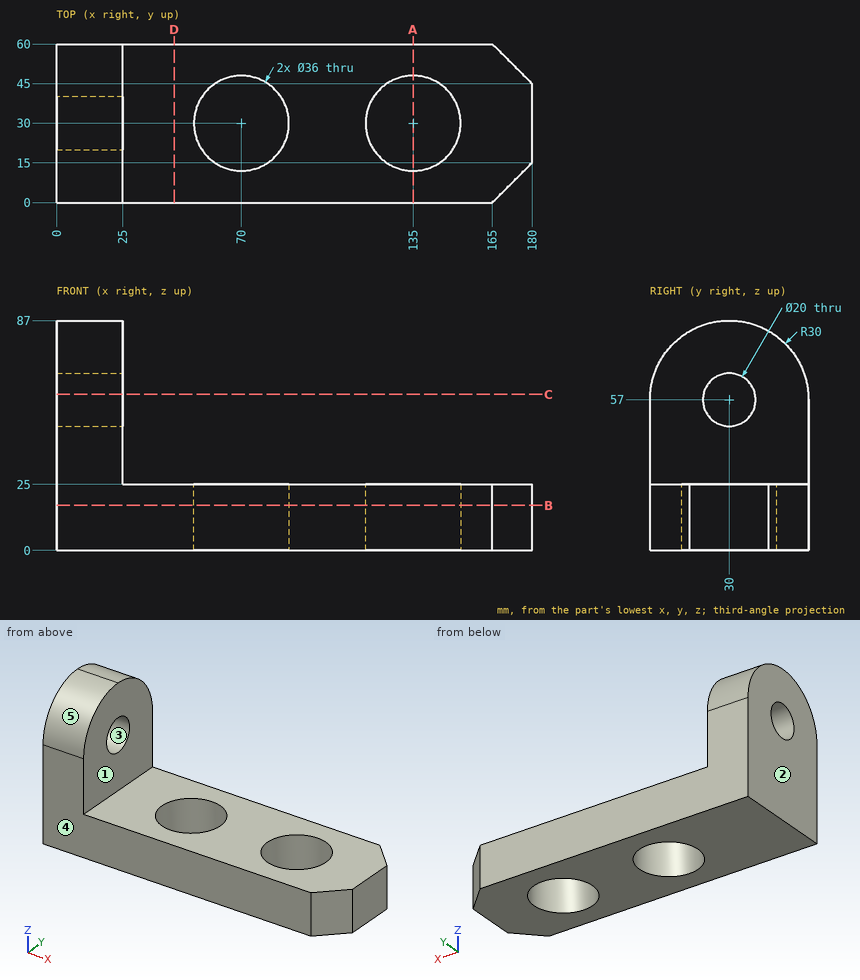
Here's the drawing with two shaded views (mm, measured from the low corner). I have some questions. A direction names the side the tool comes from. Round coordinates to 2 decimals unless told otherwise and drop trailing zeros. Loops run counter-clockwise (first coordinate to the right, second up) from the corner with the lowest first, then second, coordinate; pieces in that order, holes last. Notation, with made-up numbers: M -13.5,-31 L 26.5,-31 A31 cw 26.5,3 Z; hole C -11.75,-2 d5. An arc over 180 degrees is marked long. Answer as a JSON object with one key per item and string values. Group by question number.
Q1. Please list where these lines run through material, in increasing order: L1, parallel to X at y = 31.5, z = 10; L2, parallel to Z at x = 5.75, y = 30; L3, parallel to X at y = 3, z = 36.
Q2. We'd pull the mould along Z, two halves only. Please class the marked faces 3, 4 and 5: +Z half, -Z half, draft (parallel to the pull), parting line (faces both ways), or undercut.
Q3. Will these pins go through, and if not, where does the flat tip stop? pin 1 (10 mm diameter, centred on x = 27.5, y = 47.5, fed in from +Z); pin 2 (18 mm diameter, centred on x = 115.5, y = 43, fed in from +Z).
Q4. Imagine slicing it at A-A, the plane x = 135. Please give me the cut outline in (y, z), then the cut area to 3 significant figures.
Q5. Imagine slicing it at B-B, the plane z = 17. Please give me the cut outline in (x, y), then the cut area to 3 significant figures.
Q6. Imagine slicing it at D-D, the plane x = 44.5. Please give me the cut outline in (y, z), then the cut area to 3 significant figures.
Q7. On a 3-axis mill with a long thin cutter (end or side, diameter ignored), from which of +Z, -Z, +X, -X, +Y, -Y can I reach the whole of each face in a straight line? I mean the marked faces 1 and 2. Say none if no direction works.
Q8. Imagine slicing it at C-C, the plane z = 59. Please give me the cut outline in (x, y).
Findings:
{
 "1": {"L1": "x = 0 to 52.06, 87.94 to 117.06, 152.94 to 180", "L2": "z = 0 to 47, 67 to 87", "L3": "x = 0 to 25"},
 "2": {"face 3": "undercut", "face 4": "draft", "face 5": "+Z half"},
 "3": {"pin 1": "stops at z = 83.95", "pin 2": "stops at z = 25"},
 "4": {"outline": "M 0,0 L 12,0 L 12,25 L 0,25 Z; M 48,0 L 60,0 L 60,25 L 48,25 Z", "area": "600 mm2"},
 "5": {"outline": "M 0,0 L 165,0 L 180,15 L 180,45 L 165,60 L 0,60 Z; hole C 70,30 d36; hole C 135,30 d36", "area": "8,540 mm2"},
 "6": {"outline": "M 0,0 L 60,0 L 60,25 L 0,25 Z", "area": "1,500 mm2"},
 "7": {"face 1": "+Z, +X, +Y, -Y", "face 2": "+Z, -Z, -X, +Y, -Y"},
 "8": {"outline": "M 0,0.07 L 25,0.07 L 25,20.2 L 0,20.2 Z; M 0,39.8 L 25,39.8 L 25,59.93 L 0,59.93 Z"}
}
